Geometry: final body of the model. Coordinates: model frame, mm. A direction names the side the tool comes from. Give positions to 0.01 mm unless a question says otherwise; leave off trailing zeros. Write each loop counter-clockwise with the first axis right and the second up, starting at its lowest first coordinate (ties: lowest second). Pieces come first, ordered by that corner, then holes.
from build123d import *

# Parameters (mm, degrees)
CHANFREIN3_SIZE         = 1
ENL_V_MAT_EXTRU_1_DEPTH = 42.976183724
CHANFREIN4_SIZE         = 0.5
CHANFREIN5_SIZE         = 1.5
CHANFREIN6_SIZE         = 1
CHANFREIN7_SIZE         = 0.7
CHANFREIN2_SIZE         = 0.5


with BuildPart() as part:
    # Esquisse1 → Révolution1 (revolve)
    with BuildSketch(Plane.XY, mode=Mode.PRIVATE) as r_volution1_sk:
        Polygon((3.1, 10), (3.1, 0), (5, 0), (5, 18.12), (5, 20), (5.5, 20), (5.5, 21.22), (7.6, 21.22), (7.6, 20), (9, 20), (9, 40), (7.15, 40), (7.15, 30.27), (6.5, 30.27), (6.5, 22.77), (2.77, 22.77), (2.77, 10), align=None)
    revolve(r_volution1_sk.sketch.rotate(Axis((0, 0, 0), (0, 1, 0)), 90), axis=Axis((0, 0, 0), (0, 1, 0)))

    # Chanfrein3
    chanfrein3_edges = [part.edges().sort_by_distance(p)[0] for p in [
        (0, 40, 9),
    ]]
    chamfer(chanfrein3_edges, length=CHANFREIN3_SIZE)

    # Esquisse2 → Enlèv. mat.-Extru.1 (cut, through all)
    with BuildSketch(Plane(origin=(0, 40, 0), x_dir=(1, 0, 0), z_dir=(0, 1, 0))):
        with BuildLine():
            Line((-8, 4.123105626), (-8, -4.123105626))
            ThreePointArc((-8, -4.123105626), (-9, 0), (-8, 4.123105626))
        make_face()
        with BuildLine():
            Line((8, 4.123105626), (8, -4.123105626))
            ThreePointArc((8, -4.123105626), (9, 0), (8, 4.123105626))
        make_face()
    extrude(amount=-ENL_V_MAT_EXTRU_1_DEPTH, mode=Mode.SUBTRACT)

    # Chanfrein4
    chanfrein4_edges = [part.edges().sort_by_distance(p)[0] for p in [
        (0, 40, 7.15),
    ]]
    chamfer(chanfrein4_edges, length=CHANFREIN4_SIZE)

    # Chanfrein5
    chanfrein5_edges = [part.edges().sort_by_distance(p)[0] for p in [
        (0, 22.77, 2.77),
    ]]
    chamfer(chanfrein5_edges, length=CHANFREIN5_SIZE)

    # Chanfrein6
    chanfrein6_edges = [part.edges().sort_by_distance(p)[0] for p in [
        (0, 0, 5),
    ]]
    chamfer(chanfrein6_edges, length=CHANFREIN6_SIZE)

    # Chanfrein7
    chanfrein7_edges = [part.edges().sort_by_distance(p)[0] for p in [
        (0, 0, 3.1),
    ]]
    chamfer(chanfrein7_edges, length=CHANFREIN7_SIZE)

    # Chanfrein2
    # the kernel refuses this chamfer: 0.5 mm, written as the material it takes off along each edge
    with BuildSketch(Plane(origin=(0, 10, 0), x_dir=(0, 0, -1), z_dir=(1, 0, 0))) as chanfrein2_piece_1_section:
        Polygon((2.77 + CHANFREIN2_SIZE, 0), (2.77, CHANFREIN2_SIZE), (2.77, 0), align=None)
    chanfrein2_piece_1 = revolve(axis=Axis((0, 10, 0), (0, 1, 0)), mode=Mode.PRIVATE)
    chanfrein2_piece_1 = chanfrein2_piece_1 & Plane(origin=(0, 10.332893629, 0), x_dir=(0, 0, -1), z_dir=(0, -1, 0)) * Cylinder(3.1, 14, mode=Mode.PRIVATE)
    add(chanfrein2_piece_1, mode=Mode.SUBTRACT)
    with BuildSketch(Plane(origin=(0, 30.27, 0), x_dir=(0, 0, -1), z_dir=(1, 0, 0))) as chanfrein2_piece_2:
        Polygon((6.5, -CHANFREIN2_SIZE), (6.5 + CHANFREIN2_SIZE, 0), (6.5, 0), align=None)
    revolve(axis=Axis((0, 30.27, 0), (0, 1, 0)), mode=Mode.SUBTRACT)


solid = part.part
Q1. Pull-direction query (X, two-part tool) for faces 3 (the flat face through (8, 30, 0)), 4 (the conical face through (-0.2, 39.8, 8.2)), 5 (the cylindrical face through (1.686, 15.81, 2.198)), 6 (the flat face through (4.2, 22.77, -1.4)); classes: released by +X, released by -X, zero draft, split by the parting line, or undercut.
Filled sheet:
face 3: released by +X
face 4: split by the parting line
face 5: undercut
face 6: undercut
Q2. Section B-B on y = 36.5. Output: boundary loops of the cut face in (x, z).
Filled sheet:
outline: (-8, -4.12) arc R9 ccw to (8, -4.12) - (8, 4.12) arc R9 ccw to (-8, 4.12) - close; hole circle Ø14.3 at (0, 0)
Q3. Pin query (flat end, axial travel): P1, Ø8, axis at x = 0, z = 0, coming from the -Y side; P2, Ø1.5, axis at x = 1.5, y = 13.5, coming from the +Z side; P3, Ø5, axis at x = 0, z = 0, coming from the -Y side; P4, Ø1, axis at x = -4, y = 16.5, coming from the +Z side. Return the tip coordinate at first contact, or that it passes through.
Filled sheet:
P1: stops at y = 0
P2: stops at z = 4.94
P3: passes through
P4: stops at z = 3.57
Q4. Section A-A on y = 27.5. Output: boundary loops of the cut face in (x, z), plus the area to 3 significant figures.
Filled sheet:
outline: (-8, -4.12) arc R9 ccw to (8, -4.12) - (8, 4.12) arc R9 ccw to (-8, 4.12) - close; hole circle Ø13 at (0, 0)
area: 111 mm2
Q5. Section D-D on y = 8.5. Output: boundary loops of the cut face in (x, z), plus the area to 3 significant figures.
Filled sheet:
outline: circle Ø10 at (0, 0); hole circle Ø6.2 at (0, 0)
area: 48.3 mm2
Q6. Ray query, line 1 along X through (y, z) = (20.7, 0); line 2 along X through (y, z) = (10.15, 0); line 3 along Z through (x, y) = (0, 26.5). Return the intervals inside material, ascending.
Filled sheet:
line 1: x = -8 to -7.6, -5.5 to -2.77, 2.77 to 5.5, 7.6 to 8
line 2: x = -5 to -3.1, 3.1 to 5
line 3: z = -9 to -6.5, 6.5 to 9
Q7. Section C-C on y = 12.5. Output: boundary loops of the cut face in (x, z).
Filled sheet:
outline: circle Ø10 at (0, 0); hole circle Ø5.54 at (0, 0)
Q8. Access query for faces 1 (the cylindrical face through (5.37, 20.62, 1.19)), 2 (the flat face through (-8, 30, 0)). Directions: +Z, -Z, +X, -X, +Y, -Y. A direction counts if a zero-diameter tool reaches every point of the face in a straight line with its end or side. Return the directions, or none.
Filled sheet:
face 1: -Y
face 2: +Z, -Z, -X, +Y, -Y
